For this review, take the finished solid that the model builds, in its own axes (mm). Face numbers are marked on the shaded views. A direction names the side the tool comes from. Coordinates: 2 decimals unless noted, no trailing zeros. Write each loop counter-clockwise with the first axis right and the second up, starting at its lowest first coordinate (ties: lowest second). Pieces come first, ordered by that corner, then holes. Notation, with made-up numbers: M -10,14.5 L -4,14.5 A23 ccw -4,52.5 Z; hole C 67,31.25 d7. An arc over 180 degrees is marked long. Return JSON: item names as keys, results as strings.
```python
from build123d import *

# Parameters (mm, degrees)
SKETCH1_W             = 100
SKETCH1_H             = 40
BOSS_EXTRUDE1_DEPTH   = 3
BOSS_EXTRUDE2_DEPTH   = 0.25
BOSS_EXTRUDE21_DEPTH  = 0.5
CUT_EXTRUDE51_DEPTH   = 1
F_3_0MM_DOWEL_HOLE1_D = 3
CUT_EXTRUDE52_START   = -12
CUT_EXTRUDE52_DEPTH   = 16
SKETCH38_W            = 3
SKETCH38_H            = 0.5
SKETCH38_H_2          = 0.498463084
CUT_EXTRUDE53_DEPTH   = 0.5


with BuildPart() as part:
    # Sketch1 → Boss-Extrude1 (new body)
    with BuildSketch(Plane.XY):
        with Locations((50, -20)):
            Rectangle(SKETCH1_W, SKETCH1_H)
    extrude(amount=BOSS_EXTRUDE1_DEPTH)



with BuildPart() as body_2:
    # Sketch15 → Boss-Extrude2 (new body)
    with BuildSketch(Plane.XY.offset(3)):
        with BuildLine():
            Line((6.768599112, -11.887878533), (14.489844294, -19.704001121))
            Line((14.489844294, -19.704001121), (4.37258998, -29.821255436))
            Line((4.37258998, -29.821255436), (3, -31.193845416))
            Line((3, -31.193845416), (3, -31.476688128))
            Line((3, -31.476688128), (4.514011336, -29.962676792))
            Line((4.514011336, -29.962676792), (14.630402075, -19.846286053))
            Line((14.630402075, -19.846286053), (22.229666729, -27.538929237))
            ThreePointArc((22.229666729, -27.538929237), (28.540816637, -30.187020221), (34.868018887, -27.577516304))
            Line((34.868018887, -27.577516304), (42.552442419, -19.893092772))
            Line((42.552442419, -19.893092772), (50.282946717, -27.623597071))
            ThreePointArc((50.282946717, -27.623597071), (56.724368073, -30.291721157), (63.16578943, -27.623597071))
            Line((63.16578943, -27.623597071), (70.896293728, -19.893092772))
            Line((70.896293728, -19.893092772), (78.58071726, -27.577516304))
            ThreePointArc((78.58071726, -27.577516304), (92.175896221, -19.751671416), (78.58071726, -11.925826528))
            Line((78.58071726, -11.925826528), (70.896293728, -19.61025006))
            Line((70.896293728, -19.61025006), (63.16578943, -11.879745762))
            ThreePointArc((63.16578943, -11.879745762), (56.724368073, -9.211621675), (50.282946717, -11.879745762))
            Line((50.282946717, -11.879745762), (42.552442419, -19.61025006))
            Line((42.552442419, -19.61025006), (34.868018887, -11.925826528))
            ThreePointArc((34.868018887, -11.925826528), (28.568018887, -9.316281085), (22.268018887, -11.925826528))
            Line((22.268018887, -11.925826528), (14.631268287, -19.562577129))
            Line((14.631268287, -19.562577129), (6.910881392, -11.747323373))
            Line((6.910881392, -11.747323373), (3.163558019, -8))
            Line((3.163558019, -8), (3, -8))
            Line((3, -8), (3, -8.119279421))
            Line((3, -8.119279421), (6.768599112, -11.887878533))
        make_face()
        with BuildLine():
            Line((22.371949008, -27.398374077), (14.771826068, -19.70486206))
            Line((14.771826068, -19.70486206), (22.409440244, -12.067247885))
            ThreePointArc((22.409440244, -12.067247885), (28.568018887, -9.516281085), (34.726597531, -12.067247885))
            Line((34.726597531, -12.067247885), (42.411021063, -19.751671416))
            Line((42.411021063, -19.751671416), (34.726597531, -27.436094948))
            ThreePointArc((34.726597531, -27.436094948), (28.541427268, -29.987021153), (22.371949008, -27.398374077))
        make_face(mode=Mode.SUBTRACT)
        with BuildLine():
            Line((70.754872372, -19.751671416), (63.024368073, -27.482175714))
            ThreePointArc((63.024368073, -27.482175714), (56.724368073, -30.091721157), (50.424368073, -27.482175714))
            Line((50.424368073, -27.482175714), (42.693863775, -19.751671416))
            Line((42.693863775, -19.751671416), (50.424368073, -12.021167118))
            ThreePointArc((50.424368073, -12.021167118), (56.724368073, -9.411621675), (63.024368073, -12.021167118))
            Line((63.024368073, -12.021167118), (70.754872372, -19.751671416))
        make_face(mode=Mode.SUBTRACT)
        with BuildLine():
            Line((71.037715084, -19.751671416), (78.722138616, -12.067247885))
            ThreePointArc((78.722138616, -12.067247885), (91.962142601, -19.751671416), (78.722138616, -27.436094948))
            Line((78.722138616, -27.436094948), (71.037715084, -19.751671416))
        make_face(mode=Mode.SUBTRACT)
    extrude(amount=BOSS_EXTRUDE2_DEPTH)


with BuildPart() as part_1:
    add(part.part)

    add(body_2.part)  # Boss-Extrude21 merges body 2
    # Sketch15<71> → Boss-Extrude21 (add)
    with BuildSketch(Plane.XY.offset(3)):
        Polygon((3, -31.476688128), (3, -31.193845416), (3, -28), (0, -28), (0, -40), (100, -40), (100, 0), (0, 0), (0, -12), (3, -12), (3, -8.119279421), (3, -8), (3.163558019, -8), (94, -8), (94, -32), (3, -32), align=None)
    extrude(amount=BOSS_EXTRUDE21_DEPTH)

    # Sketch16 → Cut-Extrude51 (cut)
    with BuildSketch(Plane.XY):
        Polygon((96.84, -8), (6, -8), (6, -32), (97, -32), (97, -31.48), (100, -34.48), (100, -34.19), (97, -31.19), (97, -28), (100, -28), (100, -12), (97, -12), (97, -8.12), (100, -5.12), (100, -4.84), align=None)
    extrude(amount=CUT_EXTRUDE51_DEPTH, mode=Mode.SUBTRACT)

    # Ø3.0mm Dowel Hole1 (through all)
    with Locations(Plane.XY.offset(3.5)):
        with Locations((12, -4), (50, -4), (88, -4), (88, -36), (50, -36), (12, -36)):
            Hole(F_3_0MM_DOWEL_HOLE1_D / 2)

    # Sketch37 → Cut-Extrude52 (cut)
    with BuildSketch(Plane(origin=(0, -40, 0), x_dir=(-1, 0, 0), z_dir=(0, -1, 0)).offset(CUT_EXTRUDE52_START)):
        Polygon((0, -3.5), (-2.5, -3.5), (0, -1), align=None)
        Polygon((-100, 0), (-97.5, 0), (-100, -2.5), align=None)
    extrude(amount=-CUT_EXTRUDE52_DEPTH, mode=Mode.SUBTRACT)

    # Sketch38 → Cut-Extrude53 (cut)
    with BuildSketch(Plane.XY.offset(3.5)):
        with Locations((1.5, -9.75)):
            Rectangle(SKETCH38_W, SKETCH38_H)
        with Locations((1.5, -30.249231542)):
            Rectangle(SKETCH38_W, SKETCH38_H_2)
    extrude(amount=-CUT_EXTRUDE53_DEPTH, mode=Mode.SUBTRACT)


solid = part_1.part
```
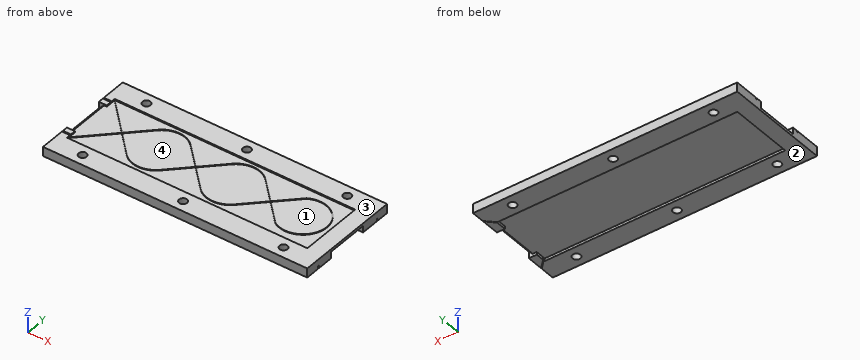
1. For the marked faces 1 and 2, list the 3-axis set-ups (+Z, -Z, +X, -X, +Y, -Y) from which the entire face can be reached by the end or side of a thin tool; tool diameter is ignored.
Checks:
{"face 1": "+Z", "face 2": "-Z, +X, -X, +Y, -Y"}
2. We need section C-C (x = 26). State the section outline as (y, z) points, plus the area to 3 significant figures.
Checks:
{"outline": "M -40,0 L -32,0 L -32,1 L -8,1 L -8,0 L 0,0 L 0,3.5 L -8,3.5 L -8,3 L -9.69,3 L -9.69,3.25 L -9.9,3.25 L -9.9,3 L -29.6,3 L -29.6,3.25 L -29.81,3.25 L -29.81,3 L -32,3 L -32,3.5 L -40,3.5 Z", "area": "104 mm2"}
3. Clearance check with flat-ended pins moving along their axes: pin 1 Ø2 at (x, z) = (27, 2.5) entering from +Y; pin 2 Ø1.8 at (x, y) = (50, -4) entering from -Z (3 decimals); pin 3 Ø11.5 at (x, y) = (47.5, -20) entering from +Z. State where each tip first meets the part, or that it passes through.
Checks:
{"pin 1": "y = 0", "pin 2": "through", "pin 3": "z = 3.25"}
4. We need section A-A (x = 12). State the section outline as (y, z) points.
Checks:
{"outline": "M -40,0 L -37.5,0 L -37.5,3.5 L -40,3.5 Z; M -34.5,0 L -32,0 L -32,1 L -8,1 L -8,0 L -5.5,0 L -5.5,3.5 L -8,3.5 L -8,3 L -16.9,3 L -16.9,3.25 L -17.18,3.25 L -17.18,3 L -22.19,3 L -22.19,3.25 L -22.48,3.25 L -22.48,3 L -32,3 L -32,3.5 L -34.5,3.5 Z; M -2.5,0 L 0,0 L 0,3.5 L -2.5,3.5 Z"}
5. Draft analysis for pull direction Y (two halves, no side actions). For the marked faces 3 and 4, state which applies: +Y half, -Y half, draft (parallel to the pull), parting line (faces both ways), or undercut.
Checks:
{"face 3": "draft", "face 4": "undercut"}
6. Wall thickness on L1, parallel to Y at x = 50, z = 2; L2, parallel to Y at x = 9, z = 0.45; L3, parallel to X at y = -29, z = 0.4: over which ranges is each line inside the solid? List them lowest first. Write a range as from..to.
Checks:
{"L1": "-40..-37.5, -34.5..-5.5, -2.5..0", "L2": "-40..-32, -8..0", "L3": "0..6, 97..100"}
7. We need section B-B (x = 84). State the section outline as (y, z) points, plus the area to 3 significant figures.
Checks:
{"outline": "M -40,0 L -32,0 L -32,1 L -8,1 L -8,0 L 0,0 L 0,3.5 L -8,3.5 L -8,3 L -10.74,3 L -10.74,3.25 L -10.95,3.25 L -10.95,3 L -28.56,3 L -28.56,3.25 L -28.76,3.25 L -28.76,3 L -32,3 L -32,3.5 L -40,3.5 Z", "area": "104 mm2"}
